from build123d import *

# Parameters (mm, degrees)
BOSS_EXTRUDE1_DEPTH      = 5.07
SKETCH2_R                = 11.585
BOSS_EXTRUDE2_DEPTH      = 3.02
CUT_EXTRUDE3_DEPTH       = 5.28
SKETCH12_R               = 4.775
CUT_EXTRUDE4_DEPTH       = 8.48
SKETCH14_R               = 2.36
BOSS_EXTRUDE5_DEPTH      = 24.51
SKETCH15_R               = 4.95
BOSS_EXTRUDE6_DEPTH      = 1.87
BOSS_EXTRUDE7_REACH      = 38.485
BOSS_EXTRUDE7_END_RADIUS = 4.95
CIRPATTERN2_COUNT        = 6
SKETCH17_R               = 1.363462741
CUT_EXTRUDE6_DEPTH       = 22.64


with BuildPart() as part:
    # Sketch1 → Boss-Extrude1 (new body)
    with BuildSketch(Plane(origin=(0, 0, 0), x_dir=(1, 0, 0), z_dir=(0, 1, 0))):
        Polygon((-3.573798166, 6.19), (-7.147596333, 0), (-3.573798166, -6.19), (3.573798166, -6.19), (7.147596333, 0), (3.573798166, 6.19), align=None)
    extrude(amount=BOSS_EXTRUDE1_DEPTH)

    # Sketch2 → Boss-Extrude2 (add)
    with BuildSketch(Plane(origin=(0, 5.07, 0), x_dir=(1, 0, 0), z_dir=(0, 1, 0))):
        with Locations(Location((0, 0, 0), (0, 0, 90))):
            Circle(SKETCH2_R)
    extrude(amount=BOSS_EXTRUDE2_DEPTH)

    # Sketch3 → Cut-Revolve1 (revolve, cut)
    with BuildSketch(Plane.XY, mode=Mode.PRIVATE) as cut_revolve1_sk:
        Polygon((10.33, 5.07), (11.585, 5.07), (11.585, 8.09), align=None)
    revolve(cut_revolve1_sk.sketch.rotate(Axis((0, 10.492775936, 0), (0, -1, 0)), 90), axis=Axis((0, 10.492775936, 0), (0, -1, 0)), mode=Mode.SUBTRACT)

    # Sketch5 → Cut-Revolve2 (revolve, cut)
    with BuildSketch(Plane.XY, mode=Mode.PRIVATE) as cut_revolve2_sk:
        Polygon((10.315, 8.09), (9.675033113, 6.55), (4.95, 6.55), (4.95, 8.27346303), (10.315, 8.27346303), align=None)
    revolve(cut_revolve2_sk.sketch.rotate(Axis((0, 10.346459419, 0), (0, -1, 0)), 90), axis=Axis((0, 10.346459419, 0), (0, -1, 0)), mode=Mode.SUBTRACT)

    # Sketch11 → Cut-Extrude3 (cut)
    with BuildSketch(Plane.XZ):
        Polygon((-2.756847535, 4.775), (-5.513695071, 0), (-2.756847535, -4.775), (2.756847535, -4.775), (5.513695071, 0), (2.756847535, 4.775), align=None)
    extrude(amount=-CUT_EXTRUDE3_DEPTH, mode=Mode.SUBTRACT)

    # Sketch12 → Cut-Extrude4 (cut)
    with BuildSketch(Plane.XZ):
        with Locations(Location((0, 0, 0), (0, 0, 90))):
            Circle(SKETCH12_R)
    extrude(amount=-CUT_EXTRUDE4_DEPTH, mode=Mode.SUBTRACT)



with BuildPart() as body_2:
    # Sketch14 → Boss-Extrude5 (new body)
    with BuildSketch(Plane(origin=(0, 8.09, 0), x_dir=(1, 0, 0), z_dir=(0, 1, 0))):
        with Locations(Location((0, 0, 0), (0, 0, 270))):
            Circle(SKETCH14_R)
    extrude(amount=BOSS_EXTRUDE5_DEPTH)


with BuildPart() as part_1:
    add(part.part)

    add(body_2.part)  # Boss-Extrude6 merges body 2
    # Sketch15 → Boss-Extrude6 (add)
    with BuildSketch(Plane(origin=(0, 8.09, 0), x_dir=(1, 0, 0), z_dir=(0, 1, 0))):
        with Locations(Location((0, 0, 0), (0, 0, 270))):
            Circle(SKETCH15_R)
    extrude(amount=BOSS_EXTRUDE6_DEPTH)

    # Boss-Extrude7: up to this cylinder (the profile starts inside it)
    boss_extrude7_end = Plane(origin=(0, 11.586667, 0), z_dir=(0, 1, 0)) * Cylinder(BOSS_EXTRUDE7_END_RADIUS, 87.87, mode=Mode.PRIVATE)
    # Sketch16 → Boss-Extrude7 (add, up to the surface)
    with BuildSketch(Plane.XY, mode=Mode.PRIVATE) as boss_extrude7_sk1:
        Polygon((0, 14.84), (-2.125, 9.96), (2.125, 9.96), align=None)
    boss_extrude7_tool1 = extrude(boss_extrude7_sk1.sketch, amount=BOSS_EXTRUDE7_REACH, mode=Mode.PRIVATE) & boss_extrude7_end
    boss_extrude7 = boss_extrude7_tool1.solids().sort_by_distance((0, 11.586667, 0))[0]
    add(boss_extrude7)

    # CirPattern2: Boss-Extrude7 ×6 about axis
    cirpattern2_axis = Axis((0, 0, 0), (0, 1, 0))
    for i in range(1, CIRPATTERN2_COUNT):
        add(boss_extrude7.rotate(cirpattern2_axis, i * 360 / CIRPATTERN2_COUNT))

    # Sketch17 → Cut-Extrude6 (cut)
    with BuildSketch(Plane(origin=(0, 32.6, 0), x_dir=(1, 0, 0), z_dir=(0, 1, 0))):
        with Locations(Location((0, 0, 0), (0, 0, 270))):
            Circle(SKETCH17_R)
    extrude(amount=-CUT_EXTRUDE6_DEPTH, mode=Mode.SUBTRACT)


solid = part_1.part
Build history of the part. All positions in model axes, mm. A direction names the side the tool comes from. Give positions to 0.01 mm unless a question says otherwise; leave off trailing zeros. Order: outer loops, then holes, each group sorted by start corner. A loop starts at its lowest first (then second) coordinate and runs counter-clockwise, first axis right, second up. Notation, with made-up numbers: M -36.75,-34.75 L 0.25,-34.75 A32 ccw 0.25,-2.75 Z; hole C -5,39 d6. An arc over 180 degrees is marked long. Use one line per item in the form item = value.
1) Drop flat-ended pins along their axis: pin 1 (4 mm diameter, centred on y = 29, z = 5.5, fed in from +X); pin 2 (5 mm diameter, centred on x = 1.5, z = -1, fed in from -Y); pin 3 (1.5 mm diameter, centred on x = 2, y = 2, fed in from +Z); pin 4 (2.5 mm diameter, centred on x = -1, z = -4, fed in from -Y). Give the stop position or say it passes through.
Calculated:
pin_1 = through
pin_2 = 8.09
pin_3 = 6.19
pin_4 = 0
2) Two-plate mould, pull along X, no slides. Class faces 1 (the face through (3.81, 12.43, -0.99)), 2 (the face through (-3.81, 12.43, 0.99)), 3 (the face through (-3, 5.28, 4)), 4 (the face through (0, 0, 5)): released by +X, released by -X, zero draft, split by the parting line, or undercut.
Calculated:
face_1 = released by +X
face_2 = released by -X
face_3 = undercut
face_4 = zero draft
3) Probe probe 1 along X at (y, z) = (22.5, 0); probe 2 along Y at (x, z) = (-2, 9.25); probe 3 along Z at (x, y) = (0.5, 27). List the from-to ranges inside material, lowest first.
Calculated:
probe_1 = -2.36 to -1.36, 1.36 to 2.36
probe_2 = 5.07 to 6.55
probe_3 = -2.31 to -1.27, 1.27 to 2.31
4) Saw through at C-C (y = 22). Give the cut face in (x, z).
Calculated:
outline = C 0,0 d4.72; hole C 0,0 d2.73
5) Saw through at A-A (y = 2). Give the cut face in (x, z) (3 decimals).
Calculated:
outline = M -7.148,0 L -3.574,-6.19 L 3.574,-6.19 L 7.148,0 L 3.574,6.19 L -3.574,6.19 Z; hole M -5.514,0 L -2.757,-4.775 L 2.757,-4.775 L 5.514,0 L 2.757,4.775 L -2.757,4.775 Z
6) Tool access for faces 5 (the face through (3.71, 12.91, 1.17)), 6 (the face through (-4.554, 9.832, 1.939)), 7 (the face through (0, 2, -6.19)), 8 (the face through (5.386, 2.5, -3.052)), 9 (the face through (4.155, 2.603, 2.354)): list every direction of +Z, -Z, +X, -X, +Y, -Y with a clear straight run to the whole face (end or side of a thin tool).
Calculated:
face_5 = +X, +Y
face_6 = +Y
face_7 = -Z, +X, -X, -Y
face_8 = -Z, +X, -Y
face_9 = -Y
7) Saw through at B-B (y = 11.5). Give the cut face in (x, z).
Calculated:
outline = M -4.82,-1.11 A4.95 ccw -3.37,-3.63 L -1.45,-2.52 L -1.45,-4.73 A4.95 ccw 1.45,-4.73 L 1.45,-2.52 L 3.37,-3.63 A4.95 ccw 4.82,-1.11 L 2.91,0 L 4.82,1.11 A4.95 ccw 3.37,3.63 L 1.45,2.52 L 1.45,4.73 A4.95 ccw -1.45,4.73 L -1.45,2.52 L -3.37,3.63 A4.95 ccw -4.82,1.11 L -2.91,0 Z; hole C 0,0 d2.73
